Build history of the part. All positions in model axes, mm. Face numbers are marked on the shaded views. Round coordinates to 2 decimals unless told otherwise and drop trailing zeros. Loops run counter-clockwise (first coordinate to the right, second up) from the corner with the lowest first, then second, coordinate; pieces in that order, holes last.
from build123d import *

# Parameters (mm, degrees)
F0_R     = 31.75
F1_DEPTH = 304.8
F2_R     = 25.4
F3_DEPTH = 304.8
F4_DEPTH = 326.39


with BuildPart() as f1:
    # F0 (on Front) → F1 (new body)
    with BuildSketch(Plane.XZ):
        Circle(F0_R)
    extrude(amount=F1_DEPTH)

    # F2 (on face) → F3 (cut)
    with BuildSketch(Plane(origin=(0, 0, 0), x_dir=(-1, 0, 0), z_dir=(0, 1, 0))):
        Circle(F2_R)
    extrude(amount=-F3_DEPTH, mode=Mode.SUBTRACT)

    # F4 (add): a face of the model
    f4_faces = [f1.faces().sort_by_distance(p)[0] for p in [
        (-30.8519743879, -304.8, 0),
    ]]
    extrude(f4_faces, amount=F4_DEPTH)


solid = f1.part
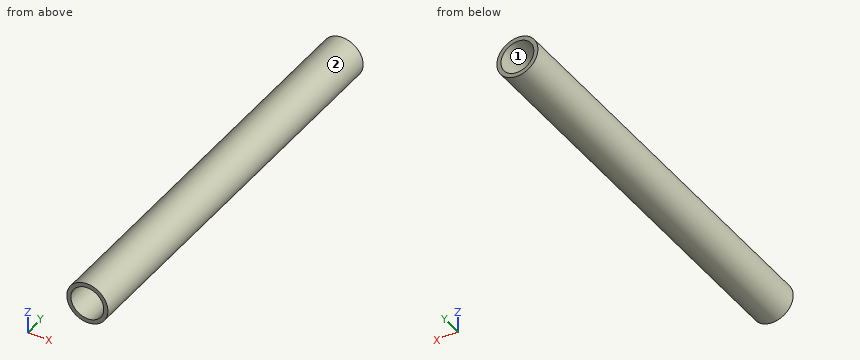
(1) Slice it at C-C on y = -372. List the corners of the cut face in (x, z).
Responses:
outline: circle Ø63.5 at (0, 0); hole circle Ø50.8 at (0, 0)
(2) Probe line 1 (Z direction, x = 0, y = -406.5); line 2 (Z direction, x = 16, y = -325); line 3 (X direction, y = -444.5, z = 18). List the from-to ranges inside material, lowest first.
Responses:
line 1: z = -31.75 to -25.4, 25.4 to 31.75
line 2: z = -27.42 to -19.73, 19.73 to 27.42
line 3: x = -26.15 to -17.92, 17.92 to 26.15
(3) Pull direction X, two halves, no side cores. Call the marked faces 1 and 2: +X half, -X half, draft (parallel to the pull), parting line (faces both ways), or undercut.
Responses:
face 1: undercut
face 2: parting line
(4) Slice it at B-B on z = 0. List the corners of the cut face in (x, y).
Responses:
outline: (-31.75, -631.19) - (-25.4, -631.19) - (-25.4, 0) - (-31.75, 0) - close; (25.4, -631.19) - (31.75, -631.19) - (31.75, 0) - (25.4, 0) - close
(5) Pin check, flat tips, straight feed: P1, Ø10, axis at y = -391, z = -16.5, coming from the -X side; P2, Ø4, axis at x = 12.5, y = -445, coming from the +Z side; P3, Ø1.5, axis at x = 6.5, y = -429.5, coming from the -Z side (3 decimals). Stop position of each tip, or through.
Responses:
P1: stops at x = -29.59
P2: stops at z = 29.96
P3: stops at z = -31.225
(6) Slice it at A-A on x = 0. List the corners of the cut face in (y, z).
Responses:
outline: (-631.19, -31.75) - (0, -31.75) - (0, -25.4) - (-631.19, -25.4) - close; (-631.19, 25.4) - (0, 25.4) - (0, 31.75) - (-631.19, 31.75) - close
